Autodesk Inventor part; units mm, degrees
ref_plane "YZ Plane" through (0, 0, 0) normal (1, 0, 0) x (0, 1, 0)
ref_plane "XZ Plane" through (0, 0, 0) normal (0, 1, 0) x (-1, 0, 0)
ref_plane "XY Plane" through (0, 0, 0) normal (0, 0, 1) x (1, 0, 0)
sketch "Sketch5" plane through (0, 0, 0) normal (0, 0, 1) x (1, 0, 0)
  line L0 (50.5, -15.6) -> (50.5, -10.6)
  line L1 (50.5, -10.6) -> (48, -10.6)
  line L2 (48, -10.6) -> (48, -12.625)
  line L3 (42, -12.625) -> (42, -2.975)
  line L4 (48, -2.975) -> (48, -5)
  line L5 (48, -5) -> (50.5, -5)
  line L6 (50.5, -5) -> (50.5, 0)
  line L7 (50.5, 0) -> (5.8, 0)
  line L8 (42, -2.975) -> (48, -2.975)
  line L9 (42, -12.625) -> (48, -12.625)
  line L10 (50.5, -15.6) -> (5.8, -15.6)
  line L11 (5.8, -15.6) -> (0, -15.6)
  line L12 (0, -15.6) -> (0, 0)
  line L13 (0, 0) -> (7.8, 0)
  line L14 (40.5, 0) -> (40.5, -15.6)
  line L15 (39.5, -15.6) -> (39.5, 0)
  line L16 (0, -45.1294) -> (0, -34.3361)
  line L17 (0, -34.3361) -> (38.5, -34.3361)
  line L18 (38.5, -34.3361) -> (38.5, -45.1294)
  line L19 (38.5, -45.1294) -> (0, -45.1294)
  line L20 (38.5, -42.4105) -> (39.5, -42.4105)
  line L21 (39.5, -42.4105) -> (39.5, -38.1261)
  line L22 (39.5, -38.1261) -> (38.5, -38.1261)
  line L23 (39.5, -42.4105) -> (39.5, -49.5786)
  line L24 (39.5, -49.5786) -> (45, -49.5786)
  line L25 (45, -49.5786) -> (45, -34.3361)
  line L26 (45, -34.3361) -> (39.5, -34.3361)
  line L27 (39.5, -34.3361) -> (39.5, -38.1261)
  point P0 (7.8, 0)
  point P1 (39, -42.4105)
  dimension "d41" = 6
  dimension "d48" = 42
  dimension "d50" = 2.5
  dimension "d63" = 44.7
  dimension "d71" = 0
  dimension "d87" = 5.6
  dimension "d88" = 9.65
  dimension "d97" = 15.6
  dimension "d122" = 1.5
  dimension "d123" = 1
  dimension "d124" = 39.5
  dimension "d125" = 38.5
  dimension "d127" = 1
  dimension "d128" = 5.5
extrude "Extrusion2" add sketch "Sketch5" along normal blind 13.5 contours L10 L14 L7 L6 L5 L4 L8 L3 L9 L2 L1 L0 | L10 L15 L7 L14 | L10 L11 L12 L13 L7 L15
fillet "Fillet2" radius 15 1 edges at (0, -15.6, 6.75)
sketch "Sketch11" plane through (0, 0, 13.5) normal (0, 0, 1) x (1, 0, 0)
  line L0 (42, -2.975) -> (48, -2.975)
  circle A0 centre (42, -2.975) radius 0.5
  line L1 (42, -12.625) -> (42, -2.975)
  circle A1 centre (42, -12.625) radius 0.5
  line L2 (48, -12.625) -> (42, -12.625)
  circle A2 centre (48, -12.625) radius 0.5
  line L3 (48, -2.975) -> (48, -5)
  circle A3 centre (48, -2.975) radius 0.5
  point P0 (0, 0)
  dimension "d99" = 1
  dimension "d100" = 1
  dimension "d101" = 1
  dimension "d102" = 1
extrude "Extrusion7" cut sketch "Sketch11" against normal through all
fillet "Rundung3" radius 5 1 edges at (0, 0, 6.75)
sketch "Skizze17" plane through (50.5, 0, 13.5) normal (0, 1, 0) x (1, 0, 0)
  line L0 (-48.97, 13.5) -> (-35.5, 13.5)
  line L1 (-46.9, 0) -> (-46.4, 0)
  line L2 (-46.4, 0) -> (-46.4, 13.5)
  line L3 (-46.4, 13.5) -> (-46.9, 13.5)
  line L4 (-46.9, 13.5) -> (-46.9, 0)
  line L5 (-44.48, 0) -> (-49.48, 0)
  line L6 (-44.48, 0) -> (-44.48, 13.5)
  point P0 (-50.5, 13.5)
  point P1 (-48.97, 0)
  point P2 (-46.65, 0)
  dimension "d140" = 0.5
  dimension "d150" = 0
  dimension "d163" = 1.92
extrude "Extrusion12" add sketch "Skizze17" along normal mid plane 3 contours L0 L2 L1 L4
sketch "Skizze18" plane through (50.5, 0, 13.5) normal (0, 1, 0) x (1, 0, 0)
  line L0 (-6.6976, 0) -> (-6.6976, 13.5)
  line L1 (-46.4, 0) -> (-46.4, 13.5)
  line L2 (0, 13.5) -> (-44.48, 13.5)
  line L3 (0, 0) -> (-44.48, 0)
  line L4 (-7.1976, 0) -> (-7.1976, 13.5)
  line L5 (-7.1976, 13.5) -> (-6.6976, 13.5)
  line L6 (-7.1976, 0) -> (-6.6976, 0)
  point P0 (-50.5, 13.5)
  dimension "d160" = 0.5
extrude "Extrusion13" add sketch "Skizze18" along normal blind 1.5
sketch "Skizze19" plane through (6.02, 0, 13.5) normal (0, 1, 0) x (1, 0, 0)
  line L0 (44.48, 13.5) -> (0, 13.5)
  line L1 (-2.3517, 13) -> (37.6723, 13)
  line L2 (37.6723, 13) -> (37.6723, 13.5)
  line L3 (37.6723, 13.5) -> (-2.3517, 13.5)
  line L4 (-2.3517, 13.5) -> (-2.3517, 13)
  line L5 (-1.92, 0) -> (-1.92, 13.5)
  point P0 (-6.02, 13.5)
  point P1 (3.0824, 14.25)
  point P2 (16.6541, 14.25)
  point P3 (24.4324, 14.25)
  dimension "d159" = 0.5
  dimension "d162" = 0
extrude "Extrusion14" add sketch "Skizze19" along normal mid plane 3
sketch "Skizze20" plane through (6.02, 0, 13.5) normal (0, 1, 0) x (1, 0, 0)
  line L0 (36.7824, 14.5) -> (36.7824, 0)
  line L1 (-2.2337, 0) -> (36.7824, 0)
  line L2 (36.7824, 0) -> (36.7824, 0.5)
  line L3 (36.7824, 0.5) -> (-2.2337, 0.5)
  line L4 (-2.2337, 0.5) -> (-2.2337, 0)
  line L5 (37.2824, 0) -> (0, 0)
  point P0 (-6.02, 13.5)
  point P1 (36.7824, 14)
  dimension "d137" = 0
  dimension "d139" = 0.5
extrude "Extrusion15" add sketch "Skizze20" along normal mid plane 3
sketch "Skizze21" plane through (6.02, 0, 0.5) normal (0, 1, 0) x (1, 0, 0)
  line L0 (8.98, 0.5) -> (44.48, 0.5)
  line L1 (31.9824, 3.6397) -> (37.2824, 3.6397)
  line L2 (37.2824, 3.6397) -> (37.2824, -19.4506)
  line L3 (37.2824, -19.4506) -> (31.9824, -19.4506)
  line L4 (31.9824, -19.4506) -> (31.9824, 3.6397)
  line L5 (36.7824, 0) -> (36.7824, -13.5)
  line L6 (37.2824, 0) -> (37.2824, -13)
  point P0 (-6.02, 0.5)
  point P1 (37.2824, -0.5)
  dimension "d152" = 5.3
  dimension "d161" = 0
extrude "Extrusion16" cut sketch "Skizze21" along normal blind 3
equation "\"l1\" = 8"
properties part number "Maria_Greifer_3D-Druck"
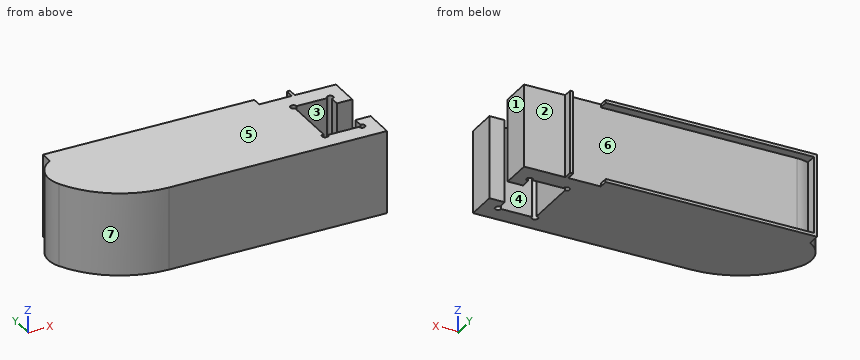
Check sheet for the modelled part. Datum: model origin and axes. Units: mm. Face numbers are marked on the shaded views. A direction names the side the tool comes from. Round coordinates to 2 decimals unless told otherwise and drop trailing zeros. Write each loop counter-clockwise with the first axis right and the second up, starting at its lowest first coordinate (ties: lowest second). Pieces come first, ordered by that corner, then holes. Notation, with made-up numbers: (40, 82) -> (69, 82) arc R25 ccw to (69, 100) -> close; hole circle Ø10 at (-24, -10.75). An arc over 180 degrees is marked (long way). One line per question, with ' | ' between items. Start each with the question number.
1. Scan lines: line 1 along Z through (x, y) = (18, 0.75); line 2 along X through (y, z) = (-13, 1.75); line 3 along X through (y, z) = (-4.75, 9.25). Record each from-to range of solid material in increasing order. Write a range as from..to.
2. Release check for a two-part mould opening along X. For the marked faces 4, 5, 6 and 7 record: +X half, -X half, draft (parallel to the pull), parting line (faces both ways), or undercut.
3. Set-up check for the marked faces 1, 2 and 3: record each of +Z, -Z, +X, -X, +Y, -Y from which the full face is reachable in a straight line by a thin tool's end or side.
4. Sectioned sample at A-A, the plane x = 47. Record the cut outline in (y, z) (3 decimals), then the cut area to 3 significant figures.
5. Sectioned sample at B-B, the plane x = 22. Record the cut outline in (y, z), then the cut area to 3 significant figures.
6. Depth check by flat-ended pin: pin 1 (6 mm diameter, centred on x = 7.5, z = 5, fed in from +Y); pin 2 (1.6 mm diameter, centred on y = 1, z = 6, fed in from -X); pin 3 (3 mm diameter, centred on y = -10, z = 11, fed in from -X). Enter the tip coordinate at first touch or a pass-through.
7. Sectioned sample at C-C, the plane x = 12. Record the cut outline in (y, z), then the cut area to 3 significant figures.
Taken from the geometry:
1) line 1: z = 0..0.5, 13..13.5 | line 2: x = 6.56..41.67, 42.33..47.67, 48.33..50.5 | line 3: x = 1.03..42, 48..50.5
2) face 4: undercut | face 5: draft | face 6: undercut | face 7: -X half
3) face 1: +Z, -Z, +X, +Y, -Y | face 2: +Z, -Z, +X, +Y | face 3: +Z, -Z
4) outline: (-15.6, 0) -> (-12.625, 0) -> (-12.625, 13.5) -> (-15.6, 13.5) -> close; (-2.975, 0) -> (0, 0) -> (0, 13.5) -> (-2.975, 13.5) -> close | area: 80.3 mm^2
5) outline: (-15.6, 0) -> (1.5, 0) -> (1.5, 0.5) -> (0, 0.5) -> (0, 13) -> (1.5, 13) -> (1.5, 13.5) -> (-15.6, 13.5) -> close | area: 212 mm^2
6) pin 1: stops at y = 0 | pin 2: stops at x = 3.6 | pin 3: stops at x = 2.25
7) outline: (-15.3, 0) -> (1.5, 0) -> (1.5, 0.5) -> (0, 0.5) -> (0, 13) -> (1.5, 13) -> (1.5, 13.5) -> (-15.3, 13.5) -> close | area: 208 mm^2
